from build123d import *

# Parameters (mm, degrees)
SKETCH_1_W          = 70
SKETCH_1_H          = 155
EXTRUDE_1_DEPTH     = 3
SKETCH_2_R          = 2
SKETCH_2_R_2        = 1.65
CUT_EXTRUDE_1_DEPTH = 3
SKETCH_3_W          = 12.5
SKETCH_3_H          = 105
SKETCH_3_H_2        = 20
CUT_EXTRUDE_2_DEPTH = 10
FILLET_1_R          = 5


with BuildPart() as part:
    # ｽｹｯﾁ1 → ﾎﾞｽ - 押し出し1 (new body)
    with BuildSketch(Plane.XY):
        Rectangle(SKETCH_1_W, SKETCH_1_H)
    extrude(amount=EXTRUDE_1_DEPTH)

    # ｽｹｯﾁ2 → ｶｯﾄ - 押し出し1 (cut)
    with BuildSketch(Plane.XY.offset(3)):
        with Locations((-17, -44.5)):
            Circle(SKETCH_2_R)
        with Locations((17, -44.5)):
            Circle(SKETCH_2_R)
        with Locations((17, -4.5)):
            Circle(SKETCH_2_R)
        with Locations((-17, -4.5)):
            Circle(SKETCH_2_R)
        with Locations((-17, 24.5)):
            Circle(SKETCH_2_R)
        with Locations((-17, 64.5)):
            Circle(SKETCH_2_R)
        with Locations((17, 64.5)):
            Circle(SKETCH_2_R)
        with Locations((17, 24.5)):
            Circle(SKETCH_2_R)
        with Locations((-30, -70)):
            Circle(SKETCH_2_R_2)
        with Locations((30, -70)):
            Circle(SKETCH_2_R_2)
        with Locations((30, 50)):
            Circle(SKETCH_2_R_2)
        with Locations((-30, 50)):
            Circle(SKETCH_2_R_2)
    extrude(amount=-CUT_EXTRUDE_1_DEPTH, mode=Mode.SUBTRACT)

    # ｽｹｯﾁ3 → ｶｯﾄ - 押し出し2 (cut)
    with BuildSketch(Plane.XY.offset(3)):
        with Locations((-28.75, -10)):
            Rectangle(SKETCH_3_W, SKETCH_3_H)
        with Locations((28.75, -10)):
            Rectangle(SKETCH_3_W, SKETCH_3_H)
        with Locations((-28.75, 67.5)):
            Rectangle(SKETCH_3_W, SKETCH_3_H_2)
        with Locations((28.75, 67.5)):
            Rectangle(SKETCH_3_W, SKETCH_3_H_2)
    extrude(amount=-CUT_EXTRUDE_2_DEPTH, mode=Mode.SUBTRACT)

    # ﾌｨﾚｯﾄ1
    fillet_1_edges = [part.edges().sort_by_distance(p)[0] for p in [
        (35, 57.5, 1.5),
        (22.5, 57.5, 1.5),
        (22.5, 77.5, 1.5),
        (35, 42.5, 1.5),
        (35, -62.5, 1.5),
        (22.5, -62.5, 1.5),
        (22.5, 42.5, 1.5),
        (-35, -62.5, 1.5),
        (-35, 42.5, 1.5),
        (-22.5, 42.5, 1.5),
        (-22.5, -62.5, 1.5),
        (-35, -77.5, 1.5),
        (35, -77.5, 1.5),
        (-35, 57.5, 1.5),
        (-22.5, 77.5, 1.5),
        (-22.5, 57.5, 1.5),
    ]]
    fillet(fillet_1_edges, radius=FILLET_1_R)


solid = part.part
Work out the finished part from the listing and answer in its coordinate system (mm). A direction names the side the tool comes from. Round coordinates to 2 decimals unless told otherwise and drop trailing zeros. Write each loop counter-clockwise with the first axis right and the second up, starting at its lowest first coordinate (ties: lowest second). Pieces come first, ordered by that corner, then holes. Notation, with made-up numbers: (33, -14) -> (77, -14) arc R21 cw to (77, 18) -> close; hole circle Ø3 at (36, -2). An arc over 180 degrees is marked (long way). Answer as CSV lines item,"result". Start each with the question number.
(1) The part is cut by section A-A, the plane y = 64.5. Give the vertices of the cut face in (x, z), then the cut area to 3 significant figures.
(2) The mould has two halves that part along Y. Classify faces 1 (the cylindrical face through (33.5, -76.07, 1.52)), 2 (the cylindrical face through (-17.434, -46.452, 1.521)), 3 (the flat face through (-22.5, 67, 2)), 4 (the flat face through (0, 77.5, 1)): +Y half, -Y half, draft (parallel to the pull), parting line (faces both ways), or undercut.
(3) The part is cut by section D-D, the plane z = 1.15. Give the number of separate pieces and of enclosed holes in the cut face, then the cut area to 3 significant figures.
(4) The part is cut by section C-C, the plane y = -70. Give the vertices of the cut face in (x, z).
(5) A tool of negligible diameter and unlimited length cuts with its end or side. For faces 5 (the flat face through (22.5, -11, 2)), 6 (the cylindrical face through (-33.57, -76, 1.52)), 7 (the flat face through (-22.5, -11, 2)), from which of +Z, -Z, +X, -X, +Y, -Y can it reach the whole face along a straight path? Write none if from no direction.
(6) Find the intervals of material crossed by probe 1 along Y at (x, z) = (-17, 0.25); probe 2 along Y at (x, z) = (30, 1.1); probe 3 along Y at (x, z) = (-29, 1.65), in increasing order.
(7) The part is cut by section B-B, the plane x = -25.5. Give the vertices of the cut face in (y, z).
(8) Each of these flat-tipped pins is pushed along its axis until it touches: pin 1 (0.8 mm diameter, centred on x = -28, z = 1, fed in from +Y); pin 2 (1 mm diameter, centred on y = -1.5, z = 2, fed in from -X). Where does it stop, or does it pass through?
Output values:
1,outline,"(-22.5, 0) -> (-19, 0) -> (-19, 3) -> (-22.5, 3) -> close; (-15, 0) -> (15, 0) -> (15, 3) -> (-15, 3) -> close; (19, 0) -> (22.5, 0) -> (22.5, 3) -> (19, 3) -> close"
1,area,"111 mm²"
2,face 1,"-Y half"
2,face 2,"undercut"
2,face 3,"draft"
2,face 4,"+Y half"
3,separate pieces,"1"
3,enclosed holes,"12"
3,area,"7,570 mm²"
4,outline,"(-35, 0) -> (-31.65, 0) -> (-31.65, 3) -> (-35, 3) -> close; (-28.35, 0) -> (28.35, 0) -> (28.35, 3) -> (-28.35, 3) -> close; (31.65, 0) -> (35, 0) -> (35, 3) -> (31.65, 3) -> close"
5,face 5,"+Z, -Z, +X"
5,face 6,"+Z, -Z, -X, -Y"
5,face 7,"+Z, -Z, -X"
6,probe 1,"y = -77.5 to -46.5, -42.5 to -6.5, -2.5 to 22.5, 26.5 to 62.5, 66.5 to 77.5"
6,probe 2,"y = -77.5 to -71.65, -68.35 to -62.5, 42.5 to 48.35, 51.65 to 57.5"
6,probe 3,"y = -77.5 to -71.31, -68.69 to -62.5, 42.5 to 48.69, 51.31 to 57.5"
7,outline,"(-77.5, 0) -> (-62.08, 0) -> (-62.08, 3) -> (-77.5, 3) -> close; (42.08, 0) -> (57.92, 0) -> (57.92, 3) -> (42.08, 3) -> close"
8,pin 1,"stops at y = 57.5"
8,pin 2,"stops at x = -22.5"
